Autodesk Inventor part; units mm, degrees
ref_plane "YZ Plane" through (0, 0, 0) normal (1, 0, 0) x (0, 1, 0)
ref_plane "XZ Plane" through (0, 0, 0) normal (0, 1, 0) x (-1, 0, 0)
ref_plane "XY Plane" through (0, 0, 0) normal (0, 0, 1) x (1, 0, 0)
sketch "Sketch5" plane through (0, 0, 0) normal (0, 0, 1) x (1, 0, 0)
  line L0 (-65, 75) -> (65, 75)
  line L1 (75, 65) -> (75, -65)
  line L2 (65, -75) -> (-65, -75)
  line L3 (-75, -65) -> (-75, 65)
  arc A0 (-65, 75) -> (-75, 65) centre (-65, 65) ccw
  arc A1 (-75, -65) -> (-65, -75) centre (-65, -65) ccw
  arc A2 (65, -75) -> (75, -65) centre (65, -65) ccw
  arc A3 (75, 65) -> (65, 75) centre (65, 65) ccw
  point P0 (0, 0)
  point P1 (-75, 75)
  point P2 (75, -75)
  point P3 (75, 75)
  dimension "d36" = 150
  dimension "d37" = 150
  dimension "d38" = 75
  dimension "d39" = 75
  dimension "d40" = 10
extrude "base" add sketch "Sketch5" along normal blind 7.5
sketch "Sketch6" plane through (0, 0, 7.5) normal (0, 0, 1) x (1, 0, 0)
  point P0 (0, 0)
  point P1 (-62.5, 62.5)
  point P2 (62.5, 62.5)
  point P3 (-62.5, -62.5)
  point P4 (62.5, -62.5)
  dimension "d43" = 125
  dimension "d44" = 125
  dimension "d45" = 62.5
  dimension "d46" = 62.5
hole "mountingHoles" at (-62.5, 62.5, 7.5) at (62.5, 62.5, 7.5) at (-62.5, -62.5, 7.5) at (62.5, -62.5, 7.5) direction (0, 0, -1) diameter 6.6 depth 8 tip angle 118 counterbore diameter 10 counterbore depth 6.5
sketch "Sketch7" plane through (0, 0, 7.5) normal (0, 0, 1) x (1, 0, 0)
  line L0 (-63, 73) -> (63, 73)
  line L1 (73, 63) -> (73, -63)
  line L2 (63, -73) -> (-63, -73)
  line L3 (-73, -63) -> (-73, 63)
  line L4 (65, 75) -> (-65, 75)
  line L5 (75, -65) -> (75, 65)
  line L6 (-65, -75) -> (65, -75)
  line L7 (-75, 65) -> (-75, -65)
  arc A0 (-63, 73) -> (-73, 63) centre (-63, 63) ccw
  arc A1 (-73, -63) -> (-63, -73) centre (-63, -63) ccw
  arc A2 (63, -73) -> (73, -63) centre (63, -63) ccw
  arc A3 (73, 63) -> (63, 73) centre (63, 63) ccw
  line L8 (-65, 75) -> (65, 75)
  line L9 (75, 65) -> (75, -65)
  line L10 (65, -75) -> (-65, -75)
  line L11 (-75, -65) -> (-75, 65)
  line L12 (-65, -75) -> (65, -75)
  arc A4 (-65, 75) -> (-75, 65) centre (-65, 65) ccw
  arc A5 (-75, -65) -> (-65, -75) centre (-65, -65) ccw
  arc A6 (65, -75) -> (75, -65) centre (65, -65) ccw
  arc A7 (75, 65) -> (65, 75) centre (65, 65) ccw
  point P0 (0, 0)
  dimension "d54" = 2
  dimension "d55" = 2
  dimension "d56" = 2
  dimension "d57" = 2
  dimension "d58" = 10
  dimension "d59" = 10
  dimension "d60" = 10
  dimension "d61" = 10
extrude "spillTray" add sketch "Sketch7" along normal blind 5
sketch "Sketch9" plane through (0, 0, 7.5) normal (0, 0, 1) x (1, 0, 0)
  circle A0 centre (0, 55) radius 1.325
  circle A1 centre (-50, 0) radius 1.325
  circle A2 centre (0, -55) radius 1.325
  circle A3 centre (50, 0) radius 1.325
  circle A4 centre (0, 0) radius 1.325
  dimension "d73" = 2.65
  dimension "d74" = 2.65
  dimension "d75" = 2.65
  dimension "d76" = 2.65
  dimension "d77" = 2.65
  dimension "d78" = 55
  dimension "d79" = 55
  dimension "d80" = 50
  dimension "d81" = 50
extrude "Extrusion5" cut sketch "Sketch9" against normal blind 2
equation "\"d55\" = d54"
equation "\"d56\" = d54"
equation "\"d57\" = d54"
equation "\"d74\" = d73"
equation "\"d75\" = d73"
equation "\"d76\" = d73"
equation "\"d77\" = d73"
properties part number "sampleHolderXYstageBase"
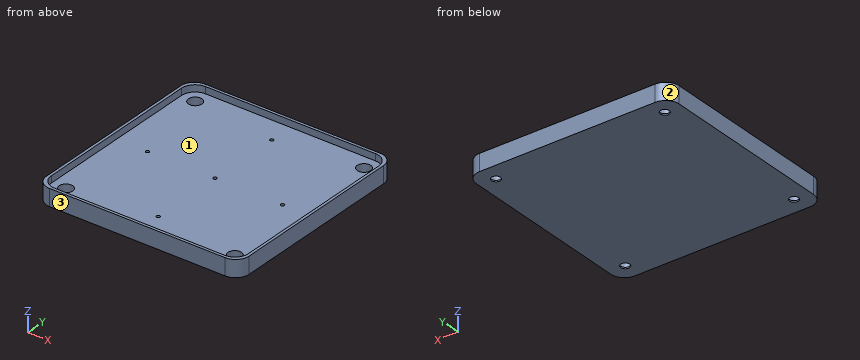
Check sheet for the modelled part. Datum: model origin and axes. Units: mm. Face numbers are marked on the shaded views. Coordinates: 2 decimals unless noted, no trailing zeros. Order: outer loops, then holes, each group sorted by start corner. A loop starts at its lowest first (then second) coordinate and runs counter-clockwise, first axis right, second up. Notation, with made-up numbers: M -30,19 L 13,19 A5 cw 13,28 Z; hole C -34,67.25 d5. An arc over 180 degrees is marked long. One line per question, with ' | ' between items. Start each with the question number.
Item 1: Mould release check, pull along Y, two halves, no side actions. Record for the marked faces 1, 2 and 3: pulls with the +Y half, pulls with the -Y half, needs draft (parallel to the pull), parting line crosses it, or undercut.
Item 2: Sectioned sample at A-A on x = -29. Record the cut outline in (y, z).
Item 3: Material ranges on line 1 (X direction, y = 62.5, z = 3); line 2 (X direction, y = -62.5, z = 0.6); line 3 (Y direction, x = 0, z = 9.5), recorded low to high.
Item 4: Gauge pin test, flat ends, axial feed: P1, Ø13, axis at x = -62.5, y = -62.5, coming from the +Z side; P2, Ø3, axis at x = 61.5, y = 60.5, coming from the +Z side; P3, Ø2, axis at x = 50, y = 0, coming from the +Z side. Record the tip position at first contact, or that the pin passes through.
Answer below:
1) face 1: undercut | face 2: pulls with the +Y half | face 3: pulls with the -Y half
2) outline: M -75,0 L 75,0 L 75,12.5 L 73,12.5 L 73,7.5 L -73,7.5 L -73,12.5 L -75,12.5 Z
3) line 1: x = -75 to -67.5, -57.5 to 57.5, 67.5 to 75 | line 2: x = -75 to -65.8, -59.2 to 59.2, 65.8 to 75 | line 3: y = -75 to -73, 73 to 75
4) P1: stops at z = 7.5 | P2: stops at z = 1 | P3: stops at z = 5.5
